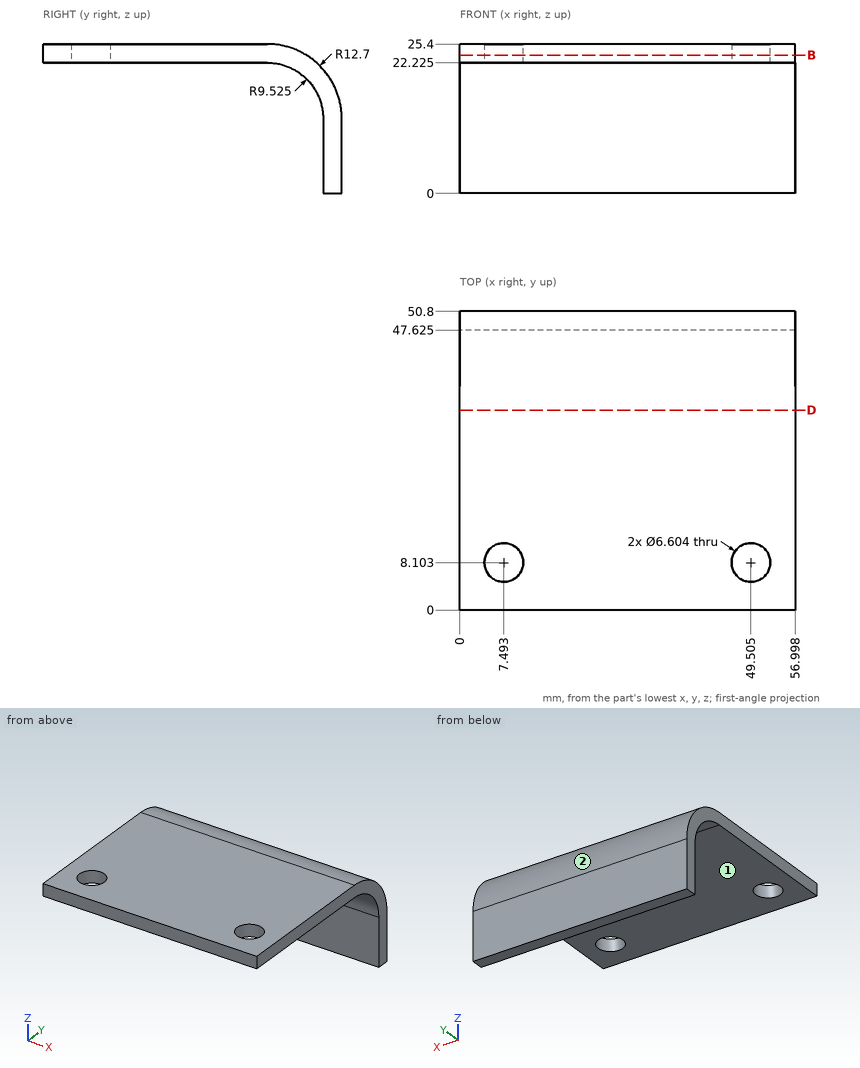
For this review, use the dimensioned drawing (mm, ordinates from the lowest corner) and the shaded views. A direction names the side the tool comes from. Give positions to 0.01 mm unless a question says otherwise; leave off trailing zeros. Write each loop counter-clockwise with the first axis right and the second up, starting at its lowest first coordinate (ties: lowest second). Pieces come first, ordered by that corner, then holes.
(1) To check wall thickness, follow L1, parallel to Z at x = 32, y = 13.5 (1 decimal); L2, parallel to Y at x = 18, z = 8.25 (1 decimal); L3, parallel to Z at x = 24, y = 44 (1 decimal). State the ranges of each line that lie inside material, in increasing order.
(2) Consider section D-D, the plane y = 34. Give the boundary of the cut face in (x, z) (1 decimal).
(3) Consider section B-B, the plane z = 23.5. Give the boundary of the cut face in (x, y) (1 decimal).
(4) For P1, Ø10, axis at x = 24.5, z = 5, coming from the -Y side (3 decimals); P2, Ø7.5, axis at x = 49.5, y = 8.1, coming from the -Z side (3 decimals); P3, Ø1.5, axis at x = 37.5, z = 18.5, coming from the -Y side (1 decimal), all flat-tipped, find the tip position at first contact; note any pin that passes through.
(5) Tool access review of the marked faces 1 and 2: name each direction out of +Z, -Z, +X, -X, +Y, -Y from which nothing blocks a thin tool from reaching the whole face with its end or side.
Returned:
1. L1: z = 22.2 to 25.4
1. L2: y = 47.6 to 50.8
1. L3: z = 20.2 to 23.9
2. outline: (0, 22.2) - (57, 22.2) - (57, 25.4) - (0, 25.4) - close
3. outline: (0, 0) - (57, 0) - (57, 44.8) - (0, 44.8) - close; hole circle Ø6.6 at (7.5, 8.1); hole circle Ø6.6 at (49.5, 8.1)
4. P1: stops at y = 47.625
4. P2: stops at z = 22.225
4. P3: stops at y = 45
5. face 1: -Z, +X, -X, -Y
5. face 2: +Z, +X, -X, +Y
